Geometry: final body of the model. Coordinates: model frame, mm. Give positions to 0.01 mm unless a question says otherwise; leave off trailing zeros. Loops run counter-clockwise (first coordinate to the right, second up) from the corner with the lowest first, then second, coordinate; pieces in that order, holes last. Notation, with made-up numbers: (70.25, -26.5) - (105.25, -26.5) arc R15 cw to (105.25, -17.5) - close; hole circle Ø2 at (-8, -9). An arc over 180 degrees is marked (long way). Answer in a Markdown table with one row per item.
from build123d import *

# Parameters (mm, degrees)
SKETCH1_R           = 11
SKETCH1_R_2         = 2.5
BOSS_EXTRUDE1_DEPTH = 22
BOSS_EXTRUDE2_START = -15
BOSS_EXTRUDE2_DEPTH = 59
CHAMFER2_SIZE       = 0.5


with BuildPart() as part:
    # Sketch1 → Boss-Extrude1 (new body)
    # profile 1 of 5: a face of its own
    with BuildSketch(Plane.XY):
        Circle(SKETCH1_R)
        Circle(SKETCH1_R_2, mode=Mode.SUBTRACT)
    # profile 2 of 5: a face of its own
    with BuildSketch(Plane.XY):
        with BuildLine():
            ThreePointArc((1.5, 2), (0, 2.5), (-1.5, 2))
            Line((-1.5, 2), (1.5, 2))
        make_face()
    # profile 3 of 5: a face of its own
    with BuildSketch(Plane.XY):
        with BuildLine():
            Line((1.5, 2), (-1.5, 2))
            ThreePointArc((-1.5, 2), (-1.118033989, -2.236067977), (2.5, 0))
            ThreePointArc((2.5, 0), (2.236067977, 1.118033989), (1.5, 2))
        make_face()
    # profile 4 of 5: a face of its own
    with BuildSketch(Plane.XY):
        with BuildLine():
            ThreePointArc((1.5, 2), (0, 2.5), (-1.5, 2))
            Line((-1.5, 2), (1.5, 2))
        make_face()
    # profile 5 of 5: a face of its own
    with BuildSketch(Plane.XY):
        with BuildLine():
            Line((1.5, 2), (-1.5, 2))
            ThreePointArc((-1.5, 2), (-1.118033989, -2.236067977), (2.5, 0))
            ThreePointArc((2.5, 0), (2.236067977, 1.118033989), (1.5, 2))
        make_face()
    extrude(amount=BOSS_EXTRUDE1_DEPTH)

    # Sketch1<3> → Boss-Extrude2 (add)
    with BuildSketch(Plane.XY.offset(BOSS_EXTRUDE2_START)):
        with BuildLine():
            ThreePointArc((1.5, 2), (0, 2.5), (-1.5, 2))
            Line((-1.5, 2), (1.5, 2))
        make_face()
        with BuildLine():
            Line((1.5, 2), (-1.5, 2))
            ThreePointArc((-1.5, 2), (-1.118033989, -2.236067977), (2.5, 0))
            ThreePointArc((2.5, 0), (2.236067977, 1.118033989), (1.5, 2))
        make_face()
    extrude(amount=BOSS_EXTRUDE2_DEPTH)

    # Chamfer2
    chamfer2_edges = [part.edges().sort_by_distance(p)[0] for p in [
        (-2.5, 0, -15),
        (-2.5, 0, 44),
    ]]
    chamfer(chamfer2_edges, length=CHAMFER2_SIZE)


solid = part.part
Q1. Cut plane C-C (y = -9). Output: boundary loops of the cut face in (x, z), and give its area (3 significant figures).
Check values:
| item | result |
|---|---|
| outline | (-6.32, 0) - (6.32, 0) - (6.32, 22) - (-6.32, 22) - close |
| area | 278 mm² |
Q2. Cut plane D-D (z = 15.5). Output: boundary loops of the cut face in (x, y).
Check values:
| item | result |
|---|---|
| outline | circle Ø22 at (0, 0) |
Q3. Material intervals for line 1 along Z through (x, y) = (-1.5, 4.5); line 2 along Y through (x, z) = (0.5, 19); line 3 along X through (y, z) = (-2, 34), sorted ascending.
Check values:
| item | result |
|---|---|
| line 1 | 0 to 22 |
| line 2 | -10.99 to 10.99 |
| line 3 | -1.5 to 1.5 |
Q4. Cut plane B-B (z = 23). Output: boundary loops of the cut face in (x, y), and give its area (3 significant figures).
Check values:
| item | result |
|---|---|
| outline | circle Ø5 at (0, 0) |
| area | 19.6 mm² |
Q5. Cut plane A-A (x = 0). Output: boundary loops of the cut face in (y, z), and give its area (4 significant figures).
Check values:
| item | result |
|---|---|
| outline | (-11, 0) - (-2.5, 0) - (-2.5, -14.5) - (-2, -15) - (2, -15) - (2.5, -14.5) - (2.5, 0) - (11, 0) - (11, 22) - (2.5, 22) - (2.5, 43.5) - (2, 44) - (-2, 44) - (-2.5, 43.5) - (-2.5, 22) - (-11, 22) - close |
| area | 668.5 mm² |
Q6. First-contact query: pin 1 (12 mm diameter, centred on y = -4.5, z = 37, fed in from -X); pin 2 (1.5 mm diameter, centred on x = 8, z = 14.5, fed in from -Y); pin 3 (12 mm diameter, centred on x = 8, y = 3, fed in from -Z). Flat tips, straight axial feed; report the tip coordinate or a pass-through.
Check values:
| item | result |
|---|---|
| pin 1 | x = -2.5 |
| pin 2 | y = -8.27 |
| pin 3 | z = 0 |
